Model file for the job. Use its own axes, mm. A direction names the side the tool comes from. Coordinates: 2 decimals unless noted, no trailing zeros. Write each loop counter-clockwise with the first axis right and the second up, starting at its lowest first coordinate (ties: lowest second). Pieces come first, ordered by that corner, then holes. Notation, with made-up numbers: M 32,-27 L 55,-27 A36 cw 55,7 Z; hole C 36.5,13 d11. An arc over 180 degrees is marked long. One line per question, with ' | ' between items. Start each with the question number.
(1) Cut at A-A (y = 6.75). Write the cut outline in (x, z), plus the area to 3 significant figures.
(2) Two-plate mould, pull along Z, no slides. Class faces 6 (the face through (-49, 11.5, 0)), 7 (the face through (29.021, 1.232, 18.125)), 8 (the face through (14.71, 1.232, 9.317)), 9 (the face through (-4, 2, -22.5)): +Z half, -Z half, draft (parallel to the pull), parting line (faces both ways), or undercut.
(3) Cut at D-D (z = 13.5). Write the cut outline in (x, y), plus the area to 3 significant figures.
(4) Tool access for faces 1 (the face through (-1, 2.5, 0)), 2 (the face through (-14.32, 1.23, -9.1)), 3 (the face through (-53, 1, -15)), 4 (the face through (53, 10, -15)), 5 (the face through (53, 1, 15)): list every direction of +Z, -Z, +X, -X, +Y, -Y with a clear straight run to the whole face (end or side of a thin tool).
(5) Cut at B-B (z = -7.5). Write the cut outline in (x, y).
(6) Cut at C-C (x = 13). Write the cut outline in (y, z), plus the area to 3 significant figures.
(7) Wall check: probe 1 along X at (y, z) = (6.75, -18.5); probe 2 along Y at (x, z) = (-48.5, 10.5); probe 3 along Z at (x, y) = (13, 1.25). Give the ranges that are in metal, low to high.
(8) Flat gauge pins, fed straight in: pin 1 Ø1.5 at (x, y) = (52, 10.5) entering from -Z; pin 2 Ø1.5 at (x, z) = (32, 17.5) entering from +Y; pin 3 Ø3.5 at (x, y) = (52.5, 1.5) entering from +Z; pin 4 Ø1.5 at (x, z) = (9.5, -9.5) entering from -Y. Where does each tip first touch, or does it go through?
from build123d import *

# Parameters (mm, degrees)
SKETCH1_W               = 12.5
SKETCH1_H               = 30
SKETCH1_W_2             = 90
SKETCH1_H_2             = 7.5
BOSS_EXTRUDE1_DEPTH     = 11.5
SKETCH2_W               = 12.5
SKETCH2_H               = 5.5
CUT_EXTRUDE1_DEPTH      = 70.604238377
CUT_EXTRUDE2_DEPTH      = 74.915492287
CUT_EXTRUDE2_DEPTH_BACK = 74.915492287
SKETCH3_W               = 80
SKETCH3_H               = 9
FILLET1_R               = 4
CUT_EXTRUDE4_DEPTH      = 10


with BuildPart() as part:
    # Sketch1 → Boss-Extrude1 (new body)
    with BuildSketch(Plane(origin=(0, 0, 0), x_dir=(1, 0, 0), z_dir=(0, 1, 0))):
        with Locations((-51.25, 0)):
            Rectangle(SKETCH1_W, SKETCH1_H)
        with Locations((0, 18.75)):
            Rectangle(SKETCH1_W_2, SKETCH1_H_2)
        Rectangle(SKETCH1_W_2, SKETCH1_H)
        with Locations((0, -18.75)):
            Rectangle(SKETCH1_W_2, SKETCH1_H_2)
        with Locations((51.25, 0)):
            Rectangle(SKETCH1_W, SKETCH1_H)
    extrude(amount=BOSS_EXTRUDE1_DEPTH)

    # Sketch2 → Cut-Extrude1 (cut, through all)
    with BuildSketch(Plane.XY.offset(15)):
        with Locations((-51.25, 5.75)):
            Rectangle(SKETCH2_W, SKETCH2_H)
    cut_extrude1 = extrude(amount=-CUT_EXTRUDE1_DEPTH, mode=Mode.SUBTRACT)

    # Mirror1: Cut-Extrude1 across plane
    add(cut_extrude1.mirror(Plane(origin=(0, 0, 0), x_dir=(0, 0, 1), z_dir=(1, 0, 0))), mode=Mode.SUBTRACT)

    # Sketch3 → Cut-Extrude2 (cut, two sides: drawn at the far end of the back side and taken through both)
    with BuildSketch(Plane.XY.offset(22.5).offset(-CUT_EXTRUDE2_DEPTH_BACK)):
        with Locations((0, 7)):
            Rectangle(SKETCH3_W, SKETCH3_H)
    extrude(amount=CUT_EXTRUDE2_DEPTH + CUT_EXTRUDE2_DEPTH_BACK, mode=Mode.SUBTRACT)

    # Fillet1
    fillet1_edges = [part.edges().sort_by_distance(p)[0] for p in [
        (-45, 10, -15),
        (45, 10, -15),
        (45, 10, 15),
        (-45, 10, 15),
        (-45, 1.5, -15),
        (-45, 1.5, 15),
        (45, 1.5, -15),
        (45, 1.5, 15),
    ]]
    fillet(fillet1_edges, radius=FILLET1_R)

    # Sketch4 → Cut-Extrude4 (cut)
    with BuildSketch(Plane.XZ):
        with BuildLine():
            Line((28.542243556, 16.981698246), (0.484736979, 1.434191182))
            ThreePointArc((0.484736979, 1.434191182), (1.9718e-05, 1.308871184), (-0.484696575, 1.434194926))
            Line((-0.484696575, 1.434194926), (-28.54169207, 16.981701989))
            ThreePointArc((-28.54169207, 16.981701989), (-29.025159296, 18.106701788), (-28.05699548, 18.856384341))
            Line((-28.05699548, 18.856384341), (28.057553721, 18.856384341))
            ThreePointArc((28.057553721, 18.856384341), (29.025718505, 18.106698049), (28.542243556, 16.981698246))
        make_face()
        with BuildLine():
            Line((30.469394666, 15.718709145), (3.68189804, 0.874682353))
            ThreePointArc((3.68189804, 0.874682353), (3.166594631, 4e-09), (3.68189804, -0.874682346))
            Line((3.68189804, -0.874682346), (30.442216306, -15.703648524))
            ThreePointArc((30.442216306, -15.703648524), (31.434112297, -15.690794907), (31.926912476, -14.829882101))
            Line((31.926912476, -14.829882101), (31.954090836, 14.843110865))
            ThreePointArc((31.954090836, 14.843110865), (31.462079818, 15.705390608), (30.469394666, 15.718709145))
        make_face()
        with BuildLine():
            Line((-3.681898037, -0.874682351), (-30.440662807, -15.70278767))
            ThreePointArc((-30.440662807, -15.70278767), (-31.432953433, -15.689701683), (-31.925359397, -14.828105319))
            Line((-31.925359397, -14.828105319), (-31.925359397, 14.828105319))
            ThreePointArc((-31.925359397, 14.828105319), (-31.432953433, 15.689701683), (-30.440662807, 15.70278767))
            Line((-30.440662807, 15.70278767), (-3.681898036, 0.874682346))
            ThreePointArc((-3.681898036, 0.874682346), (-3.166594628, -3e-09), (-3.681898037, -0.874682351))
        make_face()
        with BuildLine():
            Line((-28.057615345, -18.856727819), (28.036669402, -18.856727819))
            ThreePointArc((28.036669402, -18.856727819), (29.004796923, -18.107185608), (28.521619558, -16.982186027))
            Line((28.521619558, -16.982186027), (0.484065329, -1.434825803))
            ThreePointArc((0.484065329, -1.434825803), (-0.000739868, -1.309367606), (-0.485581416, -1.434685244))
            Line((-0.485581416, -1.434685244), (-28.542311935, -16.982045468))
            ThreePointArc((-28.542311935, -16.982045468), (-29.025779162, -18.107045266), (-28.057615345, -18.856727819))
        make_face()
    extrude(amount=-CUT_EXTRUDE4_DEPTH, mode=Mode.SUBTRACT)


solid = part.part
Filled in:
1) outline: M -45,-22.5 L -40,-22.5 L -40,22.5 L -45,22.5 Z; M 40,-22.5 L 45,-22.5 L 45,22.5 L 40,22.5 Z | area: 450 mm²
2) face 6: draft | face 7: undercut | face 8: undercut | face 9: -Z half
3) outline: M -57.5,0 L -31.93,0 L -31.93,2.5 L -40,2.5 L -40,11.5 L -57.5,11.5 L -57.5,8.5 L -45,8.5 L -45,3 L -57.5,3 Z; M -26.47,0 L -22.26,0 L -22.26,2.5 L -26.47,2.5 Z; M 22.26,0 L 26.47,0 L 26.47,2.5 L 22.26,2.5 Z; M 31.95,0 L 57.5,0 L 57.5,3 L 45,3 L 45,8.5 L 57.5,8.5 L 57.5,11.5 L 40,11.5 L 40,2.5 L 31.95,2.5 Z | area: 326 mm²
4) face 1: +Z, -Z, +Y | face 2: +Y, -Y | face 3: -Z, -X, +Y, -Y | face 4: -Z, +X, +Y, -Y | face 5: +Z, +X, +Y, -Y
5) outline: M -57.5,0 L -31.93,0 L -31.93,2.5 L -40,2.5 L -40,11.5 L -57.5,11.5 L -57.5,8.5 L -45,8.5 L -45,3 L -57.5,3 Z; M -15.64,0 L -11.43,0 L -11.43,2.5 L -15.64,2.5 Z; M 11.42,0 L 15.64,0 L 15.64,2.5 L 11.42,2.5 Z; M 31.93,0 L 57.5,0 L 57.5,3 L 45,3 L 45,8.5 L 57.5,8.5 L 57.5,11.5 L 40,11.5 L 40,2.5 L 31.93,2.5 Z
6) outline: M 0,-22.5 L 2.5,-22.5 L 2.5,-18.86 L 0,-18.86 Z; M 0,-8.38 L 2.5,-8.38 L 2.5,-6.04 L 0,-6.04 Z; M 0,6.04 L 2.5,6.04 L 2.5,8.37 L 0,8.37 Z; M 0,18.86 L 2.5,18.86 L 2.5,22.5 L 0,22.5 Z | area: 29.9 mm²
7) probe 1: -45 to -40, 40 to 45 | probe 2: 0 to 3, 8.5 to 11.5 | probe 3: -22.5 to -18.86, -8.38 to -6.04, 6.04 to 8.37, 18.86 to 22.5
8) pin 1: z = -15 | pin 2: y = 2.5 | pin 3: z = 15 | pin 4: through
